```python
from build123d import *

# Parameters (mm, degrees)
F0_W        = 23.691739887
F0_H        = 70.1130926609
F1_DEPTH    = 16.764
F2_R        = 5.08
F3_T1_DEPTH = 24.384
F3_S5_W     = 5.08
F3_S5_H     = 5.08
F3_T6_DEPTH = 5.08


# Not quite as in the source:
# - a fillet or chamfer that OpenCascade refuses, or shapes differently, is made with other operations: its cross-section is extruded or revolved along the edge and cut away or added


with BuildPart() as f1:
    # F0 (on Top) → F1 (new body)
    with BuildSketch(Plane.XY):
        with Locations((-50.7132504135, -6.1756633222)):
            Rectangle(F0_W, F0_H)
    extrude(amount=F1_DEPTH)

    # F2
    f2_edges = [f1.edges().sort_by_distance(p)[0] for p in [
        (-50.71325, 28.880883, 16.764),
        (-62.55912, -6.175663, 16.764),
        (-50.71325, -41.23221, 16.764),
        (-38.86738, -6.175663, 16.764),
        (-38.86738, -41.23221, 8.382),
        (-38.86738, 28.880883, 8.382),
        (-38.86738, -6.175663, 0),
        (-62.55912, -41.23221, 8.382),
        (-50.71325, -41.23221, 0),
    ]]
    fillet(f2_edges, radius=F2_R)

    # F3: fillet of radius 5.08 on 1 edges, made by hand

    # F3_s2 → F3_t1 (cut)
    with BuildSketch(Plane.XY.offset(-12.7)):
        with BuildLine():
            ThreePointArc((-57.479120357, 28.8808830082), (-61.0712228055, 27.3929854567), (-62.559120357, 23.8008830082))
            Line((-62.559120357, 23.8008830082), (-62.559120357, 28.8808830082))
            Line((-62.559120357, 28.8808830082), (-57.479120357, 28.8808830082))
        make_face()
    extrude(amount=F3_T1_DEPTH, mode=Mode.SUBTRACT)


with BuildPart() as f3_tool4:
    # F3_s5 → F3_t6 (new body)
    with BuildSketch(Plane.XZ.offset(-23.8008830082)):
        with Locations((-60.019120357, 14.224)):
            Rectangle(F3_S5_W, F3_S5_H)
    extrude(amount=-F3_T6_DEPTH)

    # F3_s7 → F3_t8 (revolve, cut)
    with BuildSketch(Plane(origin=(-57.479120357, 23.8008830082, 11.684), x_dir=(0.7071067812, 0, -0.7071067812), z_dir=(0.7071067812, 0, 0.7071067812))):
        with BuildLine():
            ThreePointArc((0, -5.08), (5.08, 0), (0, 5.08))
            Line((0, 5.08), (0, -5.08))
        make_face()
    revolve(axis=Axis((-57.479120357, 23.8008830082, 11.684), (0, 1, 0)), mode=Mode.SUBTRACT)


with BuildPart() as f1_1:
    add(f1.part)

    # F3_t3: cut F3_tool4
    add(f3_tool4.part, mode=Mode.SUBTRACT)


solid = f1_1.part
```
The listing builds one solid part. Answer for the finished solid, in the listing's coordinates (mm). Give positions to 0.01 mm unless a question says otherwise; leave off trailing zeros. Order: outer loops, then holes, each group sorted by start corner. A loop starts at its lowest first (then second) coordinate and runs counter-clockwise, first axis right, second up. Notation, with made-up numbers: (20.5, 73.5) -> (51.5, 73.5) arc R26 ccw to (51.5, 97.5) -> close; hole circle Ø4 at (-36, 22). An arc over 180 degrees is marked (long way). One line per item, written item: value.
1) Flat-ended cylindrical pins translate along their axes: P1, Ø4, axis at y = -11, z = 2.5, coming from the +X side; P2, Ø2, axis at x = -60, y = -31.5, coming from the +Z side. Find the tip coordinate at first contact, or state that the pin passes through.
Reported:
P1: stops at x = -38.9
P2: stops at z = 16.53
2) Find section A-A, the plane y = 13.5. Determine the outline of the cut face in (x, z).
Reported:
outline: (-62.56, 0) -> (-43.95, 0) arc R5.08 ccw to (-38.87, 5.08) -> (-38.87, 11.68) arc R5.08 ccw to (-43.95, 16.76) -> (-57.48, 16.76) arc R5.08 ccw to (-62.56, 11.68) -> close
3) Find the intervals of material crossed by line 1 (Z direction, x = -49.75, y = 24); line 2 (Y direction, x = -43.75, z = 9); line 3 (Y direction, x = -61.25, z = 2.5), in increasing order.
Reported:
line 1: z = 0 to 16.76
line 2: y = -41.23 to 28.88
line 3: y = -39.56 to 27.2
4) Find section B-B, the plane z = 3.25. Determine the outline of the cut face in (x, y).
Reported:
outline: (-62.56, -36.15) arc R5.08 ccw to (-59.31, -40.89) -> (-43.95, -40.89) arc R4.74 ccw to (-39.21, -36.15) -> (-39.21, 25.63) arc R5.08 ccw to (-43.95, 28.88) -> (-57.48, 28.88) arc R5.08 ccw to (-62.56, 23.8) -> close
5) Find section C-C, the plane x = -60.5. Determine the outline of the cut face in (y, z), plus the area to 3 significant figures.
Reported:
outline: (-40.24, 2.06) arc R5.08 ccw to (-36.15, 0) -> (27.89, 0) -> (27.89, 11.68) arc R4.08 ccw to (23.8, 15.77) -> (-36.15, 15.77) arc R4.08 ccw to (-40.24, 11.68) -> close
area: 1,060 mm^2
6) Find section D-D, the plane z = 13.5. Determine the outline of the cut face in (x, y), plus the area to 3 significant figures.
Reported:
outline: (-62.22, -36.15) arc R4.74 ccw to (-57.48, -40.9) -> (-43.95, -40.9) arc R4.74 ccw to (-39.2, -36.15) -> (-39.2, 23.8) arc R4.74 ccw to (-43.95, 28.55) -> (-57.48, 28.55) arc R4.74 ccw to (-62.22, 23.8) -> close
area: 1,580 mm^2
